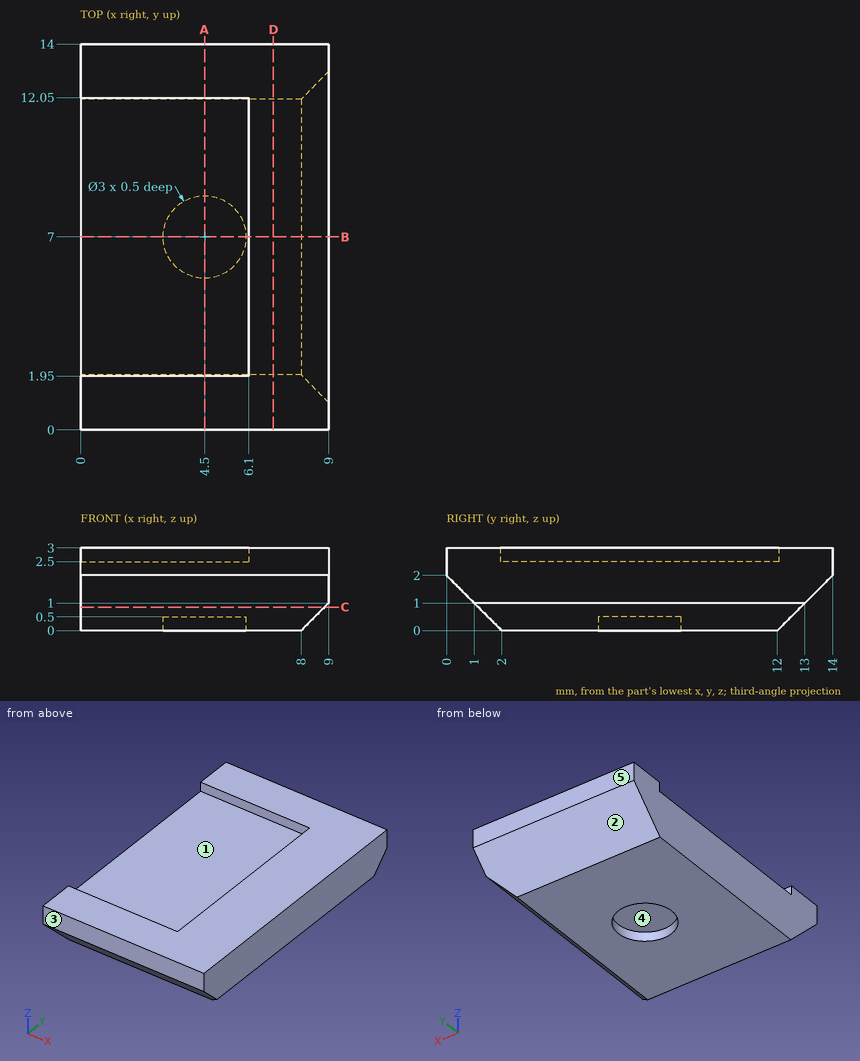
Source: three-view drawing plus pictorial views. Frame: mm from the lowest corner of the part. A direction names the side the tool comes from. Give positions to 0.01 mm unless a question says otherwise; leave off trailing zeros. Loops run counter-clockwise (first coordinate to the right, second up) from the corner with the lowest first, then second, coordinate; pieces in that order, holes last. Notation, with made-up numbers: (32.5, -33) -> (67.5, -33) arc R16 cw to (67.5, -8) -> close; hole circle Ø7 at (85.25, 13). An arc over 180 degrees is marked (long way). Use a Markdown table: item, result. Add a question column.
(1) Ray query, line 1 (Y direction, x = 1.5, z = 2.55); line 2 (Z direction, x = 2.5, y = 6); line 3 (Z direction, x = 0.5, y = 12.5). Return the intervals inside material, ascending.
(2) Section query B-B (y = 7). Output: boundary loops of the cut face in (x, z).
(3) Section query C-C (z = 0.85). Output: boundary loops of the cut face in (x, y), then the cut area to 3 significant figures.
(4) Section query A-A (x = 4.5). Output: boundary loops of the cut face in (y, z), then the cut area to 4 significant figures.
(5) First-contact query: pin 1 Ø2 at (x, y) = (5, 10.5) entering from +Z. Flat tip, straight axial feed; report the tip coordinate or a pass-through.
(6) Pull-direction query (Y, two-part tool) for the marked faces 3, 4 and 5; classes: +Y half, -Y half, draft (parallel to the pull), parting line (faces both ways), or undercut.
(7) Section query D-D (x = 7). Output: boundary loops of the cut face in (y, z), then the cut area to 3 significant figures.
(8) Access query for the marked faces 1 and 2. Directions: +Z, -Z, +X, -X, +Y, -Y. A direction counts if a zero-diameter tool reaches every point of the face in a straight line with its end or side. Return the directions, or none.
Checked values:
| question | item | result |
|---|---|---|
| 1 | line 1 | 0 to 1.95, 12.05 to 14 |
| 1 | line 2 | 0 to 2.5 |
| 1 | line 3 | 0.5 to 3 |
| 2 | outline | (0, 0) -> (3, 0) -> (3, 0.5) -> (6, 0.5) -> (6, 0) -> (8, 0) -> (9, 1) -> (9, 3) -> (6.1, 3) -> (6.1, 2.5) -> (0, 2.5) -> close |
| 3 | outline | (0, 1.15) -> (8.85, 1.15) -> (8.85, 12.85) -> (0, 12.85) -> close |
| 3 | area | 104 mm^2 |
| 4 | outline | (0, 2) -> (2, 0) -> (5.5, 0) -> (5.5, 0.5) -> (8.5, 0.5) -> (8.5, 0) -> (12, 0) -> (14, 2) -> (14, 3) -> (12.05, 3) -> (12.05, 2.5) -> (1.95, 2.5) -> (1.95, 3) -> (0, 3) -> close |
| 4 | area | 31.45 mm^2 |
| 5 | pin 1 | z = 2.5 |
| 6 | face 3 | -Y half |
| 6 | face 4 | undercut |
| 6 | face 5 | +Y half |
| 7 | outline | (0, 2) -> (2, 0) -> (12, 0) -> (14, 2) -> (14, 3) -> (0, 3) -> close |
| 7 | area | 38.0 mm^2 |
| 8 | face 1 | +Z, -X |
| 8 | face 2 | -Z, +X, -X, +Y |
